The model under review builds one solid part; all positions refer to its coordinate system, in mm. Face numbers are marked on the shaded views. A direction names the side the tool comes from. Coordinates: 2 decimals unless noted, no trailing zeros. Order: outer loops, then holes, each group sorted by start corner. A loop starts at its lowest first (then second) coordinate and runs counter-clockwise, first axis right, second up.
```python
from build123d import *

# Parameters (mm, degrees)
SKETCH3_W                    = 139.7
SKETCH3_H                    = 95.25
BASE_FLANGE1_DEPTH           = 3.175
EDGE_FLANGE1_STRIP_W         = 14.1732
EDGE_FLANGE1_STRIP_H         = 3.175
EDGE_FLANGE1_STRIP_CUT_DEPTH = 95.25
EDGE_FLANGE1_DEPTH           = 95.25
CUT_EXTRUDE2_START           = -3.175
CUT_EXTRUDE2_DEPTH           = 3.175
F_8_CLEARANCE_HOLE1_D        = 4.4958
F_1_4_CLEARANCE_HOLE1_D      = 6.7564
FILLET1_R                    = 12.7


# Read off the part's stored shape, not the designer's step: Cut-Extrude2
# Sheet-metal steps are written as plain solids
with BuildPart() as part:
    # Sketch3 → Base-Flange1 (new body)
    with BuildSketch(Plane(origin=(0, 0, 0), x_dir=(0, 0, -1), z_dir=(1, 0, 0))):
        Rectangle(SKETCH3_W, SKETCH3_H)
    extrude(amount=-BASE_FLANGE1_DEPTH)

    # Edge-Flange1 strip (across the edge) → Edge-Flange1 strip cut (cut)
    with BuildSketch(Plane(origin=(0, -47.625, -69.85), x_dir=(0, 0, 1), z_dir=(0, 1, 0))):
        with Locations((-6.35, -1.5875)):
            Rectangle(EDGE_FLANGE1_STRIP_W, EDGE_FLANGE1_STRIP_H)
    extrude(amount=EDGE_FLANGE1_STRIP_CUT_DEPTH, mode=Mode.SUBTRACT)

    # Edge-Flange1 section (across the edge) → Edge-Flange1 (add)
    with BuildSketch(Plane(origin=(0, -47.625, -69.85), x_dir=(0, 0, 1), z_dir=(0, 1, 0))):
        with BuildLine():
            Line((-3.175, 0.7366), (-3.175, 47.625))
            Line((-3.175, 47.625), (0, 47.625))
            Line((0, 47.625), (0, 0.7366))
            ThreePointArc((0, 0.7366), (0.215745145, 0.215745145), (0.7366, 0))
            Line((0.7366, 0), (0.7366, -3.175))
            ThreePointArc((0.7366, -3.175), (-2.029318885, -2.029318885), (-3.175, 0.7366))
        make_face()
    extrude(amount=EDGE_FLANGE1_DEPTH)

    # Cut-Extrude2 outline → Cut-Extrude2 (cut)
    with BuildSketch(Plane(origin=(0, 0, -73.025), x_dir=(-1, 0, 0), z_dir=(0, 0, -1)).offset(CUT_EXTRUDE2_START)):
        with BuildLine():
            ThreePointArc((-37.379054473, -20.384176045), (-44.919415432, -11.407169158), (-47.625, 0))
            Line((-47.625, 0), (-47.625, -47.625))
            Line((-47.625, -47.625), (-0.7366, -47.625))
            Line((-0.7366, -47.625), (-37.379054473, -20.384176045))
        make_face()
        with BuildLine():
            ThreePointArc((-47.625, 0), (-44.919415432, 11.407169158), (-37.379054473, 20.384176045))
            Line((-37.379054473, 20.384176045), (-0.7366, 47.625))
            Line((-0.7366, 47.625), (-47.625, 47.625))
            Line((-47.625, 47.625), (-47.625, 0))
        make_face()
    extrude(amount=CUT_EXTRUDE2_DEPTH, mode=Mode.SUBTRACT)

    # #8 Clearance Hole1 (through all)
    with Locations(Plane(origin=(0, 0, -73.025), x_dir=(-1, 0, 0), z_dir=(0, 0, -1))):
        with Locations((-25, -12.5), (-37.5, 0), (-25, 12.5), (-12.5, 0)):
            Hole(F_8_CLEARANCE_HOLE1_D / 2)

    # 1/4 Clearance Hole1 (through all)
    with Locations(Plane(origin=(0, 0, 0), x_dir=(0, 0, -1), z_dir=(1, 0, 0))):
        with Locations((-57.15, 34.925), (57.15, 34.925), (57.15, -34.925), (-57.15, -34.925)):
            Hole(F_1_4_CLEARANCE_HOLE1_D / 2)

    # Fillet1
    fillet1_edges = [part.edges().sort_by_distance(p)[0] for p in [
        (-1.5875, -47.625, 69.85),
        (-1.5875, 47.625, 69.85),
    ]]
    fillet(fillet1_edges, radius=FILLET1_R)


solid = part.part
```
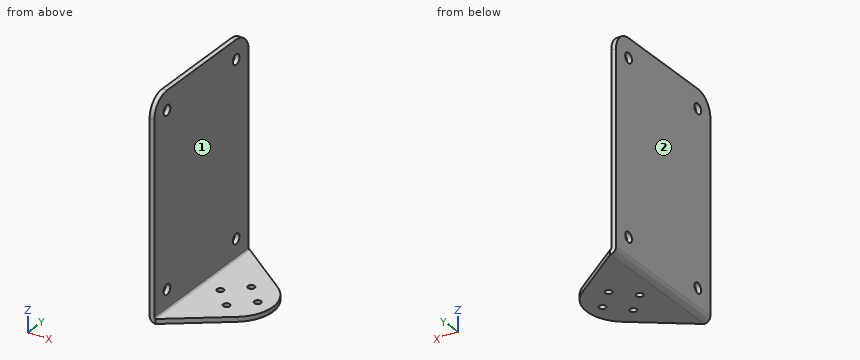
(1) Machinability: for the marked faces 1 and 2, which of the approach directions +Z, -Z, +X, -X, +Y, -Y give a long, thin tool a straight path to every point of the face, cutting with its end or side? Answer none if there is none.
A:
face 1: +Z, +X, +Y, -Y
face 2: +Z, -Z, -X, +Y, -Y
(2) We need section C-C, the plane x = 25. Write out the cut boundary in (y, z) (3 decimals), and give its area (3 significant figures).
A:
outline: (-29.587, -73.025) - (-14.748, -73.025) - (-14.748, -69.85) - (-29.587, -69.85) - close; (-10.252, -73.025) - (10.252, -73.025) - (10.252, -69.85) - (-10.252, -69.85) - close; (14.748, -73.025) - (29.587, -73.025) - (29.587, -69.85) - (14.748, -69.85) - close
area: 159 mm2
(3) We need section A-A, the plane z = -57.15. Write out the cut boundary in (x, y) (3 decimals), and give its area (3 significant figures).
A:
outline: (-3.175, -47.625) - (0, -47.625) - (0, -38.303) - (-3.175, -38.303) - close; (-3.175, -31.547) - (0, -31.547) - (0, 31.547) - (-3.175, 31.547) - close; (-3.175, 38.303) - (0, 38.303) - (0, 47.625) - (-3.175, 47.625) - close
area: 260 mm2
(4) Wall thickness on probe 1 along Y at (x, z) = (-1.45, 57.15) (3 decimals); probe 2 along Y at (x, z) = (25, -71); probe 3 along X at (y, z) = (13, 24) (3 decimals): over which ranges is each line inside the solid? List them lowest first.
A:
probe 1: y = -47.625 to -38.303, -31.547 to 31.547, 38.303 to 47.625
probe 2: y = -29.59 to -14.75, -10.25 to 10.25, 14.75 to 29.59
probe 3: x = -3.175 to 0
(5) For pin 1 Ø6 at (x, y) = (25, 12.5) entering from +Z; pin 2 Ø12 at (x, z) = (4, -2.5) entering from +Y (3 decimals); pin 3 Ø6 at (y, z) = (34.925, -57.15) entering from +X; pin 4 Ø8 at (y, z) = (-34.925, 57.15) entering from +X, all flat-tipped, find the tip position at first contact; note any pin that passes through.
A:
pin 1: stops at z = -69.85
pin 2: stops at y = 47.625
pin 3: passes through
pin 4: stops at x = 0
(6) We need section D-D, the plane x = 12.5. Write out the cut boundary in (y, z) (3 decimals).
A:
outline: (-38.88, -73.025) - (-2.248, -73.025) - (-2.248, -69.85) - (-38.88, -69.85) - close; (2.248, -73.025) - (38.88, -73.025) - (38.88, -69.85) - (2.248, -69.85) - close
(7) We need section B-B, the plane y = -12.5. Write out the cut boundary in (x, z) (3 decimals).
A:
outline: (-3.175, -69.113) arc R3.912 ccw to (0.737, -73.025) - (22.752, -73.025) - (22.752, -69.85) - (0.737, -69.85) arc R0.737 cw to (0, -69.113) - (0, 69.85) - (-3.175, 69.85) - close; (27.248, -73.025) - (44.336, -73.025) - (44.336, -69.85) - (27.248, -69.85) - close
